Autodesk Inventor part; units mm, degrees
ref_plane "YZ Plane" through (0, 0, 0) normal (1, 0, 0) x (0, 1, 0)
ref_plane "XZ Plane" through (0, 0, 0) normal (0, 1, 0) x (-1, 0, 0)
ref_plane "XY Plane" through (0, 0, 0) normal (0, 0, 1) x (1, 0, 0)
sketch "Sketch1" plane through (0, 0, 0) normal (0, 0, 1) x (1, 0, 0)
  circle A0 centre (0, 0) radius 12.5
  dimension "d0" = 25
extrude "Extrusion1" add sketch "Sketch1" along normal mid plane 142
sketch "Sketch2" plane through (0, 0, 71) normal (0, 0, 1) x (1, 0, 0)
  circle A0 centre (0, 0) radius 12.5
hole "Hole1" at (0, 0, 71) direction (0, 0, -1) diameter 8.376 depth 25 tip angle 118
mirror "Mirror1" about plane through (0, 0, 0) normal (0, 0, 1) of "Hole1"
properties part number "ADSK-MH-10013" material "Steel, Mild"
Work out the finished part from the listing and answer in its coordinate system (mm). A direction names the side the tool comes from. Give positions to 0.01 mm unless a question says otherwise; leave off trailing zeros. Loops run counter-clockwise (first coordinate to the right, second up) from the corner with the lowest first, then second, coordinate; pieces in that order, holes last. Notation, with made-up numbers: (26.25, -34) - (35.25, -34) arc R10 cw to (35.25, -18) - close; hole circle Ø9 at (7, -21.5). An arc over 180 degrees is marked (long way). One line per question, with ' | ' between items.
(1) Each of these flat-tipped pins is pushed along its axis until it touches: pin 1 Ø1.5 at (y, z) = (-4.5, 43) entering from +X; pin 2 Ø3 at (y, z) = (7, -6) entering from +X (3 decimals); pin 3 Ø1.5 at (y, z) = (8.5, 15) entering from +X; pin 4 Ø9.5 at (x, y) = (0, 0) entering from -Z. Where does it stop, or does it pass through?
Recorded:
pin 1: stops at x = 11.92 | pin 2: stops at x = 11.225 | pin 3: stops at x = 9.81 | pin 4: stops at z = -71
(2) The part is cut by section B-B (z = 34.5). Write down the section's boundary in (x, y).
Recorded:
outline: circle Ø25 at (0, 0)
(3) Straight lines are drawn through the part: probe 1 along Y at (x, z) = (0, 64.25); probe 2 along X at (y, z) = (0.5, 14.5); probe 3 along X at (y, z) = (-2.5, 54). For each, find the intervals that lie inside material, in ascending order.
Recorded:
probe 1: y = -12.5 to -4.19, 4.19 to 12.5 | probe 2: x = -12.49 to 12.49 | probe 3: x = -12.25 to -3.36, 3.36 to 12.25
(4) The part is cut by section A-A (z = -58). Write down the section's boundary in (x, y).
Recorded:
outline: circle Ø25 at (0, 0); hole circle Ø8.38 at (0, 0)
(5) A tool of negligible diameter and unlimited length cuts with its end or side. For faces 1 (the face through (2.83, 3.087, -58.325)), 2 (the face through (0, -5, -71)), 3 (the face through (-2.83, 3.087, 58.325)), from which of +Z, -Z, +X, -X, +Y, -Y can it reach the whole face along a straight path? Write none if from no direction.
Recorded:
face 1: -Z | face 2: -Z, +X, -X, +Y, -Y | face 3: +Z
(6) The mould has two halves that part along X. Classify faces 4 (the face through (0, -5, 71)), 5 (the face through (-0.72, 0.09, -43.92)), 6 (the face through (11.923, 3.755, 0.994)): +X half, -X half, draft (parallel to the pull), parting line (faces both ways), or undercut.
Recorded:
face 4: draft | face 5: undercut | face 6: parting line
(7) The part is cut by section D-D (x = -10.25). Write down the section's boundary in (y, z).
Recorded:
outline: (-7.15, -71) - (7.15, -71) - (7.15, 71) - (-7.15, 71) - close
(8) The part is cut by section C-C (x = 5.5). Write down the section's boundary in (y, z).
Recorded:
outline: (-11.22, -71) - (11.22, -71) - (11.22, 71) - (-11.22, 71) - close
